Check sheet for the modelled part. Datum: model origin and axes. Units: mm. Face numbers are marked on the shaded views. A direction names the side the tool comes from. Round coordinates to 2 decimals unless told otherwise and drop trailing zeros. Order: outer loops, then holes, each group sorted by start corner. A loop starts at its lowest first (then second) coordinate and runs counter-clockwise, first axis right, second up. Notation, with made-up numbers: (55.25, 78) -> (86.25, 78) arc R27 ccw to (86.25, 95) -> close; hole circle Ø3 at (30.5, 84.25). An arc over 180 degrees is marked (long way). Answer in a Markdown table with one row per item.
Solid Edge part; units mm, degrees
sketch "Sketch1" plane through (0, 0, 0) normal (0, -1, 0) x (1, 0, 0)
  line L0 (-63.4191, 2.9465) -> (-3.9191, 2.9465)
  line L1 (-3.9191, 2.9465) -> (-3.9191, 52.9465)
  line L2 (-3.9191, 52.9465) -> (-25.9191, 52.9465)
  line L3 (-25.9191, 52.9465) -> (-25.9191, 61.6465)
  line L4 (-25.9191, 61.6465) -> (-63.4191, 61.6465)
  dimension "D1" = 63.4191
  dimension "D2" = 3.9191
  dimension "D3" = 25.9191
  dimension "D4" = 25.9191
revolve "RevolvedProtrusion1" add sketch "Sketch1" angle 360 about axis through (-63.4191, 0, 61.6465) along (0, 0, -1)
sketch "Sketch2" plane through (-63.4191, 0, 61.6465) normal (0, 0, 1) x (1, 0, 0)
  circle A0 centre (0, 0) radius 25
extrude "Cutout1" cut sketch "Sketch2" against normal through all
sketch "Sketch3" plane through (-63.4191, 0, 52.9465) normal (0, 0, 1) x (-1, 0, 0)
  circle A0 centre (0, 0) radius 55.8511
  circle A1 centre (0, 0) radius 57.4714
extrude "Cutout2" cut sketch "Sketch3" against normal blind 20
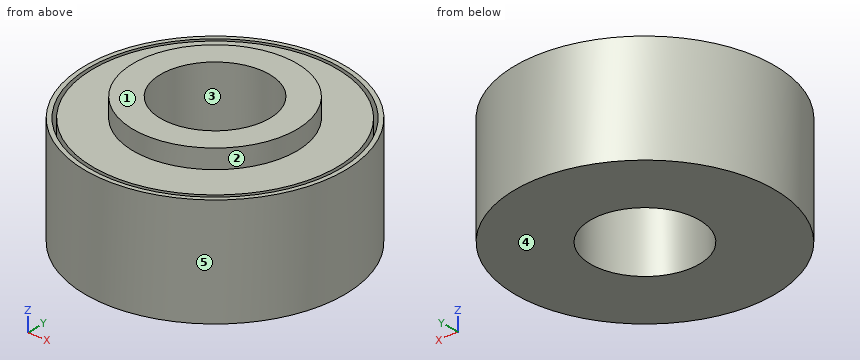
(1) Section check A-A on y = 0. Record the boundary of the cut face in (x, z), plus the area to 3 significant figures.
Solutions:
| item | result |
|---|---|
| outline | (-122.92, 2.95) -> (-88.42, 2.95) -> (-88.42, 61.65) -> (-100.92, 61.65) -> (-100.92, 52.95) -> (-119.27, 52.95) -> (-119.27, 32.95) -> (-120.89, 32.95) -> (-120.89, 52.95) -> (-122.92, 52.95) -> close; (-38.42, 2.95) -> (-3.92, 2.95) -> (-3.92, 52.95) -> (-5.95, 52.95) -> (-5.95, 32.95) -> (-7.57, 32.95) -> (-7.57, 52.95) -> (-25.92, 52.95) -> (-25.92, 61.65) -> (-38.42, 61.65) -> close |
| area | 3,600 mm^2 |
(2) Draft check along X on the marked faces 3, 4 and 5. Enter one of: pulls with the +X half, pulls with the -X half, needs draft (parallel to the pull), parting line crosses it, or undercut.
Solutions:
| item | result |
|---|---|
| face 3 | undercut |
| face 4 | needs draft |
| face 5 | parting line crosses it |
(3) Section check C-C on x = -58.5. Record the boundary of the cut face in (y, z), plus the area to 3 significant figures.
Solutions:
| item | result |
|---|---|
| outline | (-59.3, 2.95) -> (-24.51, 2.95) -> (-24.51, 61.65) -> (-37.18, 61.65) -> (-37.18, 52.95) -> (-55.63, 52.95) -> (-55.63, 32.95) -> (-57.26, 32.95) -> (-57.26, 52.95) -> (-59.3, 52.95) -> close; (24.51, 2.95) -> (59.3, 2.95) -> (59.3, 52.95) -> (57.26, 52.95) -> (57.26, 32.95) -> (55.63, 32.95) -> (55.63, 52.95) -> (37.18, 52.95) -> (37.18, 61.65) -> (24.51, 61.65) -> close |
| area | 3,630 mm^2 |
(4) Section check D-D on z = 58. Record the boundary of the cut face in (x, y), plus the area to 3 significant figures.
Solutions:
| item | result |
|---|---|
| outline | circle Ø75 at (-63.42, 0); hole circle Ø50 at (-63.42, 0) |
| area | 2,450 mm^2 |
(5) Depth check by flat-ended pin: pin 1 Ø1 at (x, y) = (-103, 16.5) entering from +Z; pin 2 Ø10 at (y, z) = (-6, 53.5) entering from +X; pin 3 Ø10 at (y, z) = (26, 11) entering from +X. Enter the tip coordinate at first touch or a pass-through.
Solutions:
| item | result |
|---|---|
| pin 1 | z = 52.95 |
| pin 2 | x = -3.93 |
| pin 3 | x = -7.75 |
(6) Scan lines: probe 1 along Y at (x, z) = (-46.5, 50) (3 decimals); probe 2 along Y at (x, z) = (-53, 50.5); probe 3 along X at (y, z) = (41, 52). Record each from-to range of solid material in increasing order. Write a range as from..to.
Solutions:
| item | result |
|---|---|
| probe 1 | -57.044..-54.925, -53.227..-18.405, 18.405..53.227, 54.925..57.044 |
| probe 2 | -58.58..-56.52, -54.87..-22.73, 22.73..54.87, 56.52..58.58 |
| probe 3 | -106.54..-103.69, -101.34..-25.49, -23.15..-20.3 |
(7) Tool access check on the marked faces 1 and 2. Record the directions out of +Z, -Z, +X, -X, +Y, -Y that give a thin tool (end or side, any length) a straight path to the whole face; none if there is none.
Solutions:
| item | result |
|---|---|
| face 1 | +Z, +X, -X, +Y, -Y |
| face 2 | +Z |
(8) Section check B-B on z = 43.5. Record the boundary of the cut face in (x, y), plus the area to 3 significant figures.
Solutions:
| item | result |
|---|---|
| outline | circle Ø119 at (-63.42, 0); circle Ø111.7 at (-63.42, 0); hole circle Ø114.94 at (-63.42, 0); hole circle Ø50 at (-63.42, 0) |
| area | 8,580 mm^2 |
